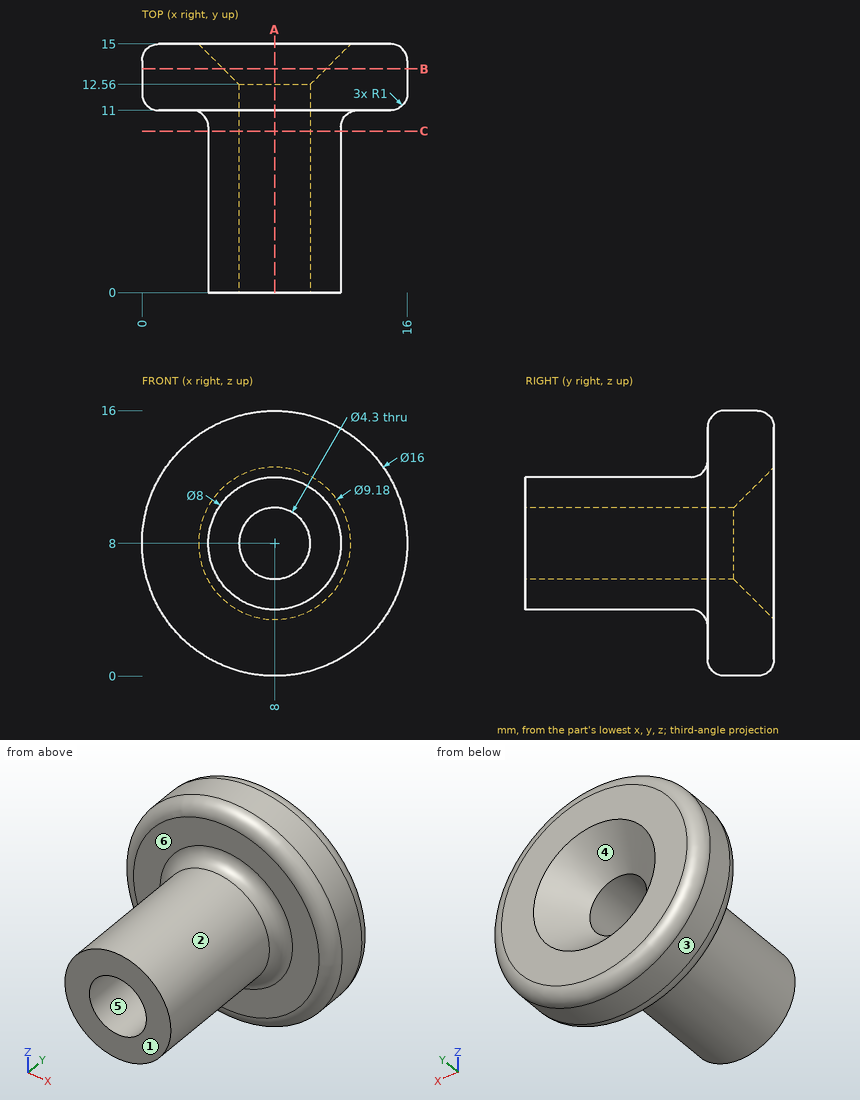
Source: three-view drawing plus pictorial views. Frame: mm from the lowest corner of the part. A direction names the side the tool comes from. Coordinates: 2 decimals unless noted, no trailing zeros. Loops run counter-clockwise (first coordinate to the right, second up) from the corner with the lowest first, then second, coordinate; pieces in that order, holes last. Notation, with made-up numbers: M 45.5,74.5 L 100.5,74.5 A28 ccw 100.5,102.5 Z; hole C 72,46.25 d9. An arc over 180 degrees is marked long. Use CSV: the item, a comma, the result in double quotes.
(1) Line query: line 1 (Z direction, x = 8, y = 8.5); line 2 (Y direction, x = 7, z = 14); line 3 (Z direction, x = 11.75, y = 14.5). Output: solid intervals per line, ascending. Write a range as [from, to].
Answers follow:
line 1,"[4, 5.85], [10.15, 12]"
line 2,"[11, 15]"
line 3,"[1.09, 6.37], [9.63, 14.91]"
(2) Contact query for flat-ended pins moving along their axis: pin 1 (6 mm diameter, centred on y = 2.5, z = 10, fed in from +X); pin 2 (1.5 mm diameter, centred on y = 11.5, z = 6, fed in from -X); pin 3 (1.5 mm diameter, centred on x = 7, z = 11.5, fed in from +Y). Output: stop coordinate, or through.
Answers follow:
pin 1,"x = 12"
pin 2,"x = 0.12"
pin 3,"y = 14.8"
(3) Draft query along X for the marked faces 3, 4, 5 and 6. Return one class per face: pulls with the +X half, pulls with the -X half, needs draft (parallel to the pull), parting line crosses it, or undercut.
Answers follow:
face 3,"parting line crosses it"
face 4,"undercut"
face 5,"undercut"
face 6,"needs draft"
(4) Cut plane C-C on y = 9.75. Return loops of the section in (x, z), and give its area (3 significant figures).
Answers follow:
outline,"C 8,8 d8; hole C 8,8 d4.3"
area,"35.7 mm²"
(5) Reachability of the marked faces 1 and 2 from +Z, -Z, +X, -X, +Y, -Y: full face, straight path, thin tool, end or side. Return the list, or none.
Answers follow:
face 1,"+Z, -Z, +X, -X, -Y"
face 2,"-Y"
(6) Cut plane A-A on x = 8. Return loops of the section in (y, z).
Answers follow:
outline,"M 0,4 L 10,4 A1 cw 11,3 L 11,1 A1 ccw 12,0 L 14,0 A1 ccw 15,1 L 15,3.41 L 12.56,5.85 L 0,5.85 Z; M 0,10.15 L 12.56,10.15 L 15,12.59 L 15,15 A1 ccw 14,16 L 12,16 A1 ccw 11,15 L 11,13 A1 cw 10,12 L 0,12 Z"
(7) Cut plane B-B on y = 13.5. Return loops of the section in (x, z), and give its area (3 significant figures).
Answers follow:
outline,"C 8,8 d16; hole C 8,8 d6.18"
area,"171 mm²"
